Answer from the drawing. Dimensions are ordinates in mm from the lowest x, y and z of the part. A direction names the side the tool comes from. Coordinates: 2 decimals unless noted, no trailing zeros. Write each loop counter-clockwise with the first axis right and the second up, starting at its lowest first coordinate (ties: lowest second). Pieces come first, ordered by that corner, then holes. Notation, with made-up numbers: M 80,-18.5 L 104,-18.5 A18 ccw 104,15.5 Z; hole C 11.25,-10.75 d7. An arc over 180 degrees is marked long. Put each result on its own line as item: value. Start each with the question number.
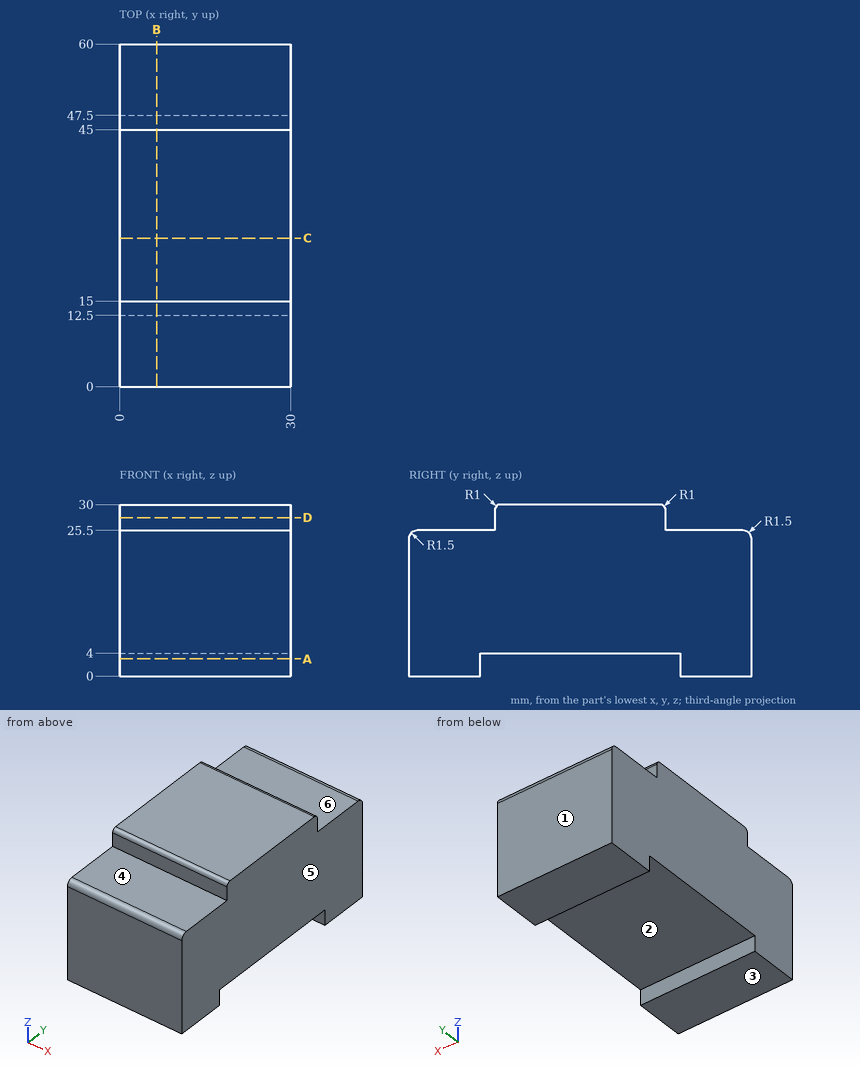
1) Given pin 1 Ø11 at (x, y) = (21.5, 5.5) entering from +Z; pin 2 Ø9 at (x, y) = (19.5, 29.5) entering from -Z, each flat-ended and moving along its own axis, determine where each tip first touches the part or whether it passes through.
2) Determine the mould class of the marked faces 1, 2 and 3 for opening direction Y: +Y half, -Y half, draft (parallel to the pull), parting line (faces both ways), or undercut.
3) For the marked faces 4, 5 and 6, determine the directions among +Z, -Z, +X, -X, +Y, -Y from which every point of the face is accessible in a straight line to the end or side of a thin tool.
4) Straight lines are drawn through the part: probe 1 along Z at (x, y) = (7, 34.5); probe 2 along Y at (x, z) = (4, 27.75); probe 3 along Z at (x, y) = (20.75, 14). For each, find the intervals that lie inside material, in ascending order.
5) A cutting plane is placed at A-A on z = 3. Write down the section's boundary in (x, y), then the cut area to 3 significant figures.
6) A cutting plane is placed at B-B on x = 6.5. Write down the section's boundary in (y, z), then the cut area to 3 significant figures.
7) A cutting plane is placed at D-D on z = 27.75. Write down the section's boundary in (x, y).
8) A cutting plane is placed at C-C on y = 26. Write down the section's boundary in (x, z), then the cut area to 3 significant figures.
Answers follow:
1. pin 1: stops at z = 25.5
1. pin 2: stops at z = 4
2. face 1: +Y half
2. face 2: undercut
2. face 3: draft
3. face 4: +Z, +X, -X, -Y
3. face 5: +Z, -Z, +X, +Y, -Y
3. face 6: +Z, +X, -X, +Y
4. probe 1: z = 4 to 30
4. probe 2: y = 15 to 45
4. probe 3: z = 4 to 25.5
5. outline: M 0,0 L 30,0 L 30,12.5 L 0,12.5 Z; M 0,47.5 L 30,47.5 L 30,60 L 0,60 Z
5. area: 750 mm²
6. outline: M 0,0 L 12.5,0 L 12.5,4 L 47.5,4 L 47.5,0 L 60,0 L 60,24 A1.5 ccw 58.5,25.5 L 45,25.5 L 45,29 A1 ccw 44,30 L 16,30 A1 ccw 15,29 L 15,25.5 L 1.5,25.5 A1.5 ccw 0,24 Z
6. area: 1,520 mm²
7. outline: M 0,15 L 30,15 L 30,45 L 0,45 Z
8. outline: M 0,4 L 30,4 L 30,30 L 0,30 Z
8. area: 780 mm²
